```python
from build123d import *

# Parameters (mm, degrees)
F0_R     = 3.175
F1_DEPTH = 3.048


# Not quite as in the source:
# - a feature names something its author has since deleted; it is built from what else it names


with BuildPart() as f1:
    # F0 (on Front) → F1 (new body)
    with BuildSketch(Plane.XZ):
        with BuildLine():
            ThreePointArc((-9.524828548, 63.1542134468), (-6.7149560856, 56.455996051), (0, 53.6863635294))
            ThreePointArc((0, 53.6863635294), (6.7149544249, 56.4559944002), (9.5248285199, 63.1542087637))
            ThreePointArc((9.5248285199, 63.1542087637), (9.5249571299, 63.1827860179), (9.525, 63.2113635294))
            ThreePointArc((9.525, 63.2113635294), (-0.0285751699, 72.7363206663), (-9.524828548, 63.1542134468))
        make_face()
        with BuildLine():
            ThreePointArc((3.175, 63.2113635294), (2.2450640303, 60.9662994992), (0, 60.0363635294))
            ThreePointArc((0, 60.0363635294), (-2.2450640303, 65.4564275597), (3.175, 63.2113635294))
        make_face(mode=Mode.SUBTRACT)
        with BuildLine():
            ThreePointArc((9.5248285199, 63.1542087637), (6.7149544249, 56.4559944002), (0, 53.6863635294))
            Line((0, 53.6863635294), (0, 48.9365635294))
            Line((0, 48.9365635294), (0, 28.2863635294))
            ThreePointArc((0, 28.2863635294), (9.7569068314, 24.9340786537), (15.3931294165, 16.2930116029))
            Line((15.3931294165, 16.2930116029), (9.5248285199, 63.1542087637))
        make_face()
        with BuildLine():
            Line((0, 48.9365635294), (0, 53.6863635294))
            ThreePointArc((0, 53.6863635294), (-6.7149560856, 56.455996051), (-9.524828548, 63.1542134468))
            Line((-9.524828548, 63.1542134468), (-15.7471542329, 14.4220247552))
            ThreePointArc((-15.7471542329, 14.4220247552), (-10.4903855516, 24.3263723829), (0, 28.2863635294))
            Line((0, 28.2863635294), (0, 48.9365635294))
        make_face()
        with Locations((-3.175, 48.9365635294)):
            Circle(F0_R, mode=Mode.SUBTRACT)
        with BuildLine():
            ThreePointArc((15.3931294165, 16.2930116029), (9.7569068314, 24.9340786537), (0, 28.2863635294))
            Line((0, 28.2863635294), (0, 15.5863635294))
            ThreePointArc((0, 15.5863635294), (2.2450640303, 14.6564275597), (3.175, 12.4113635294))
            ThreePointArc((3.175, 12.4113635294), (2.2450640303, 10.1662994992), (0, 9.2363635294))
            Line((0, 9.2363635294), (0, -3.4636364706))
            ThreePointArc((0, -3.4636364706), (9.6997269009, -0.1556935265), (15.3571050572, 8.3895543266))
            Line((15.3571050572, 8.3895543266), (15.8749636535, 12.445334128))
            Line((15.8749636535, 12.445334128), (15.3931294165, 16.2930116029))
        make_face()
        with BuildLine():
            Line((0, 15.5863635294), (0, 28.2863635294))
            ThreePointArc((0, 28.2863635294), (-10.4903855516, 24.3263723829), (-15.7471542329, 14.4220247552))
            Line((-15.7471542329, 14.4220247552), (-14.8425870633, 6.7799130706))
            ThreePointArc((-14.8425870633, 6.7799130706), (-9.017104551, -0.6541426038), (0, -3.4636364706))
            Line((0, -3.4636364706), (0, 9.2363635294))
            ThreePointArc((0, 9.2363635294), (-3.175, 12.4113635294), (0, 15.5863635294))
        make_face()
        with BuildLine():
            ThreePointArc((0, -3.4636364706), (-9.017104551, -0.6541426038), (-14.8425870633, 6.7799130706))
            Line((-14.8425870633, 6.7799130706), (-7.8824732142, -52.0216543038))
            ThreePointArc((-7.8824732142, -52.0216543038), (-5.9333689967, -45.8161571108), (0, -43.1511364706))
            Line((0, -43.1511364706), (0, -3.4636364706))
        make_face()
        with BuildLine():
            ThreePointArc((15.3571050572, 8.3895543266), (9.6997269009, -0.1556935265), (0, -3.4636364706))
            Line((0, -3.4636364706), (0, -43.1511364706))
            ThreePointArc((0, -43.1511364706), (5.6126600757, -45.4759763949), (7.9375, -51.0886364706))
            Line((7.9375, -51.0886364706), (36.5125, -51.0886364706))
            ThreePointArc((36.5125, -51.0886364706), (38.8373399243, -45.4759763949), (44.45, -43.1511364706))
            Line((44.45, -43.1511364706), (17.8060374021, -43.1511364706))
            ThreePointArc((17.8060374021, -43.1511364706), (11.8390009683, -40.4545215548), (9.9198625623, -34.1939973287))
            Line((9.9198625623, -34.1939973287), (15.3571050572, 8.3895543266))
        make_face()
        with BuildLine():
            ThreePointArc((0, -43.1511364706), (-5.9333689967, -45.8161571108), (-7.8824732142, -52.0216543038))
            ThreePointArc((-7.8824732142, -52.0216543038), (-5.2724793598, -57.0220054673), (0, -59.0261364706))
            ThreePointArc((0, -59.0261364706), (5.6126600757, -56.7012965462), (7.9375, -51.0886364706))
            Line((7.9375, -51.0886364706), (3.175, -51.0886364706))
            ThreePointArc((3.175, -51.0886364706), (-2.2450640303, -53.3337005008), (0, -47.9136364706))
            Line((0, -47.9136364706), (0, -43.1511364706))
        make_face()
        with BuildLine():
            ThreePointArc((7.9375, -51.0886364706), (5.6126600757, -45.4759763949), (0, -43.1511364706))
            Line((0, -43.1511364706), (0, -47.9136364706))
            ThreePointArc((0, -47.9136364706), (2.2450640303, -48.8435724403), (3.175, -51.0886364706))
            Line((3.175, -51.0886364706), (7.9375, -51.0886364706))
        make_face()
        with BuildLine():
            ThreePointArc((7.9375, -51.0886364706), (5.6126600757, -56.7012965462), (0, -59.0261364706))
            Line((0, -59.0261364706), (44.45, -59.0261364706))
            ThreePointArc((44.45, -59.0261364706), (38.8373399243, -56.7012965462), (36.5125, -51.0886364706))
            Line((36.5125, -51.0886364706), (7.9375, -51.0886364706))
        make_face()
        with BuildLine():
            ThreePointArc((36.5125, -51.0886364706), (38.8373399243, -56.7012965462), (44.45, -59.0261364706))
            ThreePointArc((44.45, -59.0261364706), (50.0626600757, -56.7012965462), (52.3875, -51.0886364706))
            ThreePointArc((52.3875, -51.0886364706), (50.0626600757, -45.4759763949), (44.45, -43.1511364706))
            ThreePointArc((44.45, -43.1511364706), (38.8373399243, -45.4759763949), (36.5125, -51.0886364706))
        make_face()
        with BuildLine():
            ThreePointArc((47.625, -51.0886364706), (44.45, -54.2636364706), (41.275, -51.0886364706))
            ThreePointArc((41.275, -51.0886364706), (44.45, -47.9136364706), (47.625, -51.0886364706))
        make_face(mode=Mode.SUBTRACT)
    extrude(amount=F1_DEPTH)


solid = f1.part
```
Design review of the part built by this model. Coordinates are the model's own, in mm. A direction names the side the tool comes from. Give positions to 0.01 mm unless a question says otherwise; leave off trailing zeros. Order: outer loops, then holes, each group sorted by start corner. A loop starts at its lowest first (then second) coordinate and runs counter-clockwise, first axis right, second up. Notation, with made-up numbers: (67.25, -37) -> (75.25, -37) arc R7 ccw to (75.25, -25) -> close; hole circle Ø7 at (12.5, -22.75). An arc over 180 degrees is marked (long way). Write item = value, one per line. Start each with the question number.
(1) We need section C-C on z = 36. Write out the cut boundary in (x, y), plus the area to 3 significant figures.
(2) For faces 1 (the face through (31, -2, -43.151)), 2 (the face through (3, -3.048, 8)), list the 3-axis set-ups (+Z, -Z, +X, -X, +Y, -Y) from which the entire face can be reached by the end or side of a thin tool; tool diameter is ignored.
(3) Mouldability with a two-part tool opening along X and no side actions: class faces 3 (the face through (22, -2, -59.026)), 4 (the face through (11.902, -1.503, -40.525)), 5 (the face through (-1.468, -1.503, 51.614)) as +X half, -X half, draft (parallel to the pull), parting line (faces both ways), or undercut.
(4) We need section A-A on y = -0.55. State how many separate pieces and enclosed holes the cut face has, plus the area to 3 significant figures.
(5) To check wall thickness, follow line 1 along X through (y, z) = (-2.85, -52.5); line 2 along X through (y, z) = (-0.95, -52) (3 decimals); line 3 along Z through (x, y) = (26, -0.85). State the ranges of each line that lie inside material, in increasing order.
(6) For pin 1 (1.5 mm diameter, centred on y = -1.5, z = -24.5, fed in from -X), flat-tipped, find the tip position at first contact; note if it passes through.
(7) We need section B-B on x = 28. Write out the cut boundary in (y, z).
Numbers:
q1.outline = (-12.99, -3.05) -> (12.93, -3.05) -> (12.93, 0) -> (-12.99, 0) -> close
q1.area = 79.0 mm^2
q2.face_1 = +Z, +X, +Y, -Y
q2.face_2 = +Z, -Z, +X, -X, -Y
q3.face_3 = draft
q3.face_4 = +X half
q3.face_5 = undercut
q4.separate_pieces = 1
q4.enclosed_holes = 5
q4.area = 3,580 mm^2
q5.line_1 = -7.81 to -2.84, 2.84 to 41.61, 47.29 to 52.26
q5.line_2 = -7.885 to -3.041, 3.041 to 41.409, 47.491 to 52.335
q5.line_3 = -59.03 to -43.15
q6.pin_1 = -11.23
q7.outline = (-3.05, -59.03) -> (0, -59.03) -> (0, -43.15) -> (-3.05, -43.15) -> close
